```python
from build123d import *

# Parameters (mm, degrees)
SKETCH_3_R      = 7.5
EXTRUDE_3_DEPTH = 30
SKETCH_4_W      = 20
SKETCH_4_H      = 20
EXTRUDE_4_DEPTH = 45


with BuildPart() as part:
    # ｽｹｯﾁ3 → ﾎﾞｽ - 押し出し3 (new body)
    with BuildSketch(Plane(origin=(0, 0, 0), x_dir=(1, 0, 0), z_dir=(0, 1, 0))):
        with Locations(Location((0, 0, 0), (0, 0, 270))):
            Circle(SKETCH_3_R)
    extrude(amount=EXTRUDE_3_DEPTH)

    # ｽｹｯﾁ4 → ﾎﾞｽ - 押し出し4 (add)
    with BuildSketch(Plane.XZ):
        Rectangle(SKETCH_4_W, SKETCH_4_H)
    extrude(amount=EXTRUDE_4_DEPTH)


solid = part.part
```
The listing builds one solid part. Answer for the finished solid, in the listing's coordinates (mm). A direction names the side the tool comes from. Give positions to 0.01 mm unless a question says otherwise; leave off trailing zeros. Order: outer loops, then holes, each group sorted by start corner. A loop starts at its lowest first (then second) coordinate and runs counter-clockwise, first axis right, second up. Notation, with made-up numbers: (21.5, 27.5) -> (29.5, 27.5) arc R36 ccw to (29.5, 66.5) -> close; hole circle Ø5 at (1, 86). An arc over 180 degrees is marked (long way). One line per item, written item: value.
1) Flat-ended cylindrical pins translate along their axes: P1, Ø8, axis at y = 5, z = -3, coming from the +X side; P2, Ø1.5, axis at y = 13, z = 6, coming from the +X side; P3, Ø3, axis at x = 6.5, y = 0.5, coming from the +Z side. Find the tip coordinate at first contact, or state that the pin passes through.
Reported:
P1: stops at x = 7.5
P2: stops at x = 5.36
P3: stops at z = 10
2) Find section C-C, the plane y = 5. Determine the outline of the cut face in (x, z).
Reported:
outline: circle Ø15 at (0, 0)
3) Find section A-A, the plane z = 0. Determine the outline of the cut face in (x, y), plus the area to 3 significant figures.
Reported:
outline: (-10, -45) -> (10, -45) -> (10, 0) -> (7.5, 0) -> (7.5, 30) -> (-7.5, 30) -> (-7.5, 0) -> (-10, 0) -> close
area: 1,350 mm^2
4) Find section B-B, the plane x = 0. Determine the outline of the cut face in (y, z).
Reported:
outline: (-45, -10) -> (0, -10) -> (0, -7.5) -> (30, -7.5) -> (30, 7.5) -> (0, 7.5) -> (0, 10) -> (-45, 10) -> close
5) Find the intervals of material crossed by line 1 (Y direction, x = 8.5, z = -0.5); line 2 (Z direction, x = 1.5, y = 5.5); line 3 (Z direction, x = -4.5, y = 10), in increasing order.
Reported:
line 1: y = -45 to 0
line 2: z = -7.35 to 7.35
line 3: z = -6 to 6
6) A tool of negligible diameter and unlimited length cuts with its end or side. For faces 1 (the flat face through (4, 0, 7)), 2 (the flat face through (-10, -22, 0)), from which of +Z, -Z, +X, -X, +Y, -Y can it reach the whole face along a straight path? Write none if from no direction.
Reported:
face 1: +Y
face 2: +Z, -Z, -X, +Y, -Y
